```python
from build123d import *

# Parameters (mm, degrees)
SKETCH1_R           = 3
BOSS_EXTRUDE1_DEPTH = 2


with BuildPart() as part:
    # Sketch1 → Boss-Extrude1 (new, symmetric)
    with BuildSketch(Plane(origin=(0, 0, 0), x_dir=(0, 0, -1), z_dir=(1, 0, 0))):
        with BuildLine():
            Line((-8, 0), (-6, 50))
            ThreePointArc((-6, 50), (0, 56), (6, 50))
            Line((6, 50), (8, 0))
            ThreePointArc((8, 0), (0, -8), (-8, 0))
        make_face()
        Circle(SKETCH1_R, mode=Mode.SUBTRACT)
        with BuildLine():
            Line((2, 50), (2, 30))
            ThreePointArc((2, 30), (0, 28), (-2, 30))
            Line((-2, 30), (-2, 50))
            ThreePointArc((-2, 50), (0, 52), (2, 50))
        make_face(mode=Mode.SUBTRACT)
    extrude(amount=BOSS_EXTRUDE1_DEPTH, both=True)


solid = part.part
```
Part model, mm, in its own coordinate system. A direction names the side the tool comes from. Round coordinates to 2 decimals unless told otherwise and drop trailing zeros. Write each loop counter-clockwise with the first axis right and the second up, starting at its lowest first coordinate (ties: lowest second). Pieces come first, ordered by that corner, then holes. Notation, with made-up numbers: M 85,-7.75 L 135,-7.75 A18 ccw 135,10.25 Z; hole C 38.25,17 d6. An arc over 180 degrees is marked long. One line per question, with ' | ' between items.
(1) Probe line 1 along Y through (x, z) = (1, 0); line 2 along Z through (x, y) = (-1.25, 35); line 3 along Z through (x, y) = (-0.1, 43). List the from-to ranges inside material, lowest first.
Answer key:
line 1: y = -8 to -3, 3 to 28, 52 to 56 | line 2: z = -6.6 to -2, 2 to 6.6 | line 3: z = -6.28 to -2, 2 to 6.28
(2) Saw through at C-C on x = -0.75. Write the cut outline in (y, z), then the cut area to 3 significant figures.
Answer key:
outline: M 0,-8 L 50,-6 A6 ccw 50,6 L 0,8 A8 ccw Z; hole C 0,0 d6; hole M 30,-2 L 50,-2 A2 ccw 50,2 L 30,2 A2 ccw Z | area: 736 mm^2
(3) Saw through at A-A on y = 41. Write the cut outline in (x, z).
Answer key:
outline: M -2,-6.36 L 2,-6.36 L 2,-2 L -2,-2 Z; M -2,2 L 2,2 L 2,6.36 L -2,6.36 Z
(4) 3-axis set-ups, long thin cutter, end or side, ignore diameter. For faces 1 (the face through (-2, 17, 0)), 2 (the face through (0, 40, 2)): which of +Z, -Z, +X, -X, +Y, -Y reach the whole face in a straight line?
Answer key:
face 1: +Z, -Z, -X, +Y, -Y | face 2: +X, -X
(5) Saw through at D-D on y = 34. Write the cut outline in (x, z), then the cut area to 3 significant figures.
Answer key:
outline: M -2,-6.64 L 2,-6.64 L 2,-2 L -2,-2 Z; M -2,2 L 2,2 L 2,6.64 L -2,6.64 Z | area: 37.1 mm^2
(6) Saw through at B-B on z = 0. Write the cut outline in (x, y), then the cut area to 3 significant figures.
Answer key:
outline: M -2,-8 L 2,-8 L 2,-3 L -2,-3 Z; M -2,3 L 2,3 L 2,28 L -2,28 Z; M -2,52 L 2,52 L 2,56 L -2,56 Z | area: 136 mm^2
(7) Two-plate mould, pull along Y, no slides. Class faces 3 (the face through (0, 56, 0)), 4 (the face through (0, 0, 3)), 5 (the face through (2, 17, 0)): released by +Y, released by -Y, zero draft, split by the parting line, or undercut.
Answer key:
face 3: released by +Y | face 4: undercut | face 5: zero draft
(8) Pin check, flat tips, straight feed: pin 1 (1.2 mm diameter, centred on x = -0.5, y = 37, fed in from +Z); pin 2 (2 mm diameter, centred on x = -0.5, y = 36, fed in from -Z); pin 3 (1.5 mm diameter, centred on x = 1, z = -1.5, fed in from -Y); pin 4 (5.5 mm diameter, centred on y = 0, z = 0, fed in from -X). Stop position of each tip, or through.
Answer key:
pin 1: stops at z = 6.54 | pin 2: stops at z = -6.6 | pin 3: stops at y = -7.96 | pin 4: passes through
